Source: CAD feature listing. Evaluate the final solid. Frame: model axes, mm. Face numbers are marked on the shaded views. Round coordinates to 2 decimals unless told otherwise and drop trailing zeros. Order: outer loops, then holes, each group sorted by start corner. A loop starts at its lowest first (then second) coordinate and runs counter-clockwise, first axis right, second up. Notation, with made-up numbers: (57.25, 76) -> (75.25, 76) arc R24 cw to (75.25, 89) -> close; hole circle Ø6 at (-33, -31). An arc over 180 degrees is marked (long way). Use a Markdown table: item, result. Add a question column.
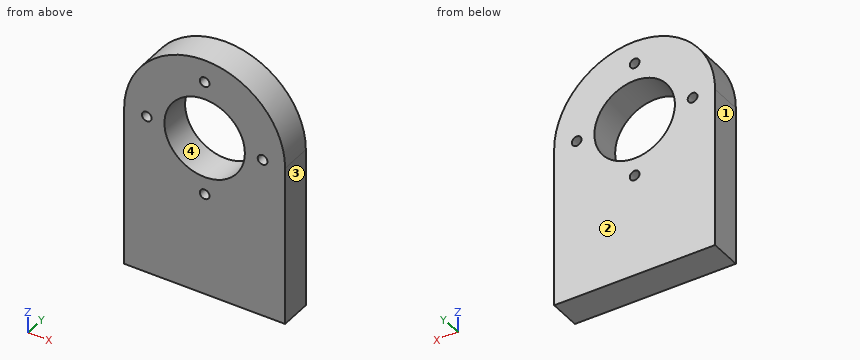
```python
from build123d import *

# Parameters (mm, degrees)
F0_W     = 200
F0_H     = 40
F0_R     = 50
F1_DEPTH = 40
F2_D     = 12.1


with BuildPart() as f1:
    # F0 (on Front) → F1 (new body)
    with BuildSketch(Plane.XZ):
        with Locations((0, 20)):
            Rectangle(F0_W, F0_H)
        with BuildLine():
            Line((-100, 200), (-100, 40))
            Line((-100, 40), (100, 40))
            Line((100, 40), (100, 200))
            ThreePointArc((100, 200), (0, 300), (-100, 200))
        make_face()
        with Locations((0, 200)):
            Circle(F0_R, mode=Mode.SUBTRACT)
    extrude(amount=F1_DEPTH)

    # F2 (through all)
    with Locations(Plane(origin=(0, 0, 0), x_dir=(1, 0, 0), z_dir=(0, 1, 0))):
        with Locations((0, -272), (-72, -200), (0, -128), (72, -200)):
            Hole(F2_D / 2)


solid = f1.part
```
1) Section B-B on z = 128. Output: boundary loops of the cut face in (x, y), then the cut area to 3 significant figures.
2) Draft query along X for the marked faces 1, 2, 3 and 4. Return one class per face: pulls with the +X half, pulls with the -X half, needs draft (parallel to the pull), parting line crosses it, or undercut.
3) Section C-C on y = -12.5. Output: boundary loops of the cut face in (x, z), then the cut area to 3 significant figures.
4) Section A-A on x = 0. Output: boundary loops of the cut face in (y, z), then the cut area to 3 significant figures.
5) Section D-D on x = -72. Output: boundary loops of the cut face in (y, z), then the cut area to 3 significant figures.
6) First-contact query: pin 1 Ø5 at (x, y) = (-78.5, -29.5) entering from -Z; pin 2 Ø11 at (x, z) = (-72, 200) entering from +Y; pin 3 Ø10 at (x, y) = (-49.5, -28.5) entering from +Z; pin 4 Ø2 at (x, y) = (-62.5, -10) entering from +Z. Flat tips, straight axial feed; report the tip coordinate or a pass-through.
7) Line query: probe 1 along Z at (x, y) = (0, -23); probe 2 along X at (y, z) = (-26.5, 127.5); probe 3 along Z at (x, y) = (-72, -30). Output: solid intervals per line, ascending. Write a range as from..to.
Conclusion:
| question | item | result |
|---|---|---|
| 1 | outline | (-100, -40) -> (-6.05, -40) -> (-6.05, 0) -> (-100, 0) -> close; (6.05, -40) -> (100, -40) -> (100, 0) -> (6.05, 0) -> close |
| 1 | area | 7,520 mm^2 |
| 2 | face 1 | pulls with the -X half |
| 2 | face 2 | needs draft |
| 2 | face 3 | pulls with the +X half |
| 2 | face 4 | undercut |
| 3 | outline | (-100, 0) -> (100, 0) -> (100, 200) arc R100 ccw to (-100, 200) -> close; hole circle Ø12.1 at (-72, 200); hole circle Ø100 at (0, 200); hole circle Ø12.1 at (0, 128); hole circle Ø12.1 at (0, 272); hole circle Ø12.1 at (72, 200) |
| 3 | area | 47,400 mm^2 |
| 4 | outline | (-40, 0) -> (0, 0) -> (0, 121.95) -> (-40, 121.95) -> close; (-40, 134.05) -> (0, 134.05) -> (0, 150) -> (-40, 150) -> close; (-40, 250) -> (0, 250) -> (0, 265.95) -> (-40, 265.95) -> close; (-40, 278.05) -> (0, 278.05) -> (0, 300) -> (-40, 300) -> close |
| 4 | area | 7,030 mm^2 |
| 5 | outline | (-40, 0) -> (0, 0) -> (0, 193.95) -> (-40, 193.95) -> close; (-40, 206.05) -> (0, 206.05) -> (0, 269.4) -> (-40, 269.4) -> close |
| 5 | area | 10,300 mm^2 |
| 6 | pin 1 | stops at z = 0 |
| 6 | pin 2 | passes through |
| 6 | pin 3 | stops at z = 289.55 |
| 6 | pin 4 | stops at z = 278.85 |
| 7 | probe 1 | z = 0..121.95, 134.05..150, 250..265.95, 278.05..300 |
| 7 | probe 2 | x = -100..-6.03, 6.03..100 |
| 7 | probe 3 | z = 0..193.95, 206.05..269.4 |
